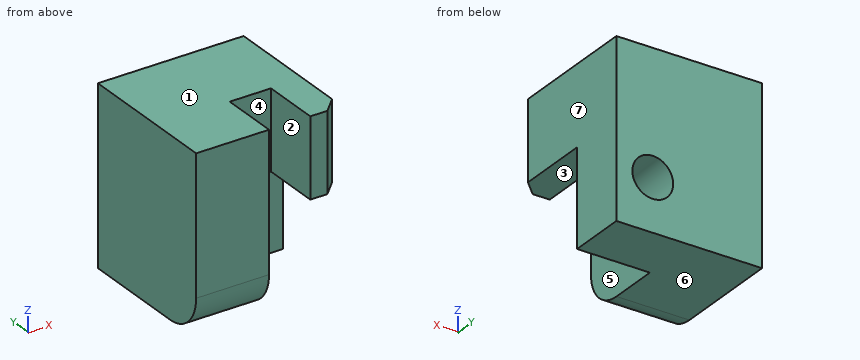
from build123d import *

# Parameters (mm, degrees)
F0_W     = 127
F0_H     = 152.4
F1_DEPTH = 127
F2_W     = 63.5
F2_H     = 83.7710094534
F3_DEPTH = 76.2
F4_R     = 17.78
F5_DEPTH = 50.8
F6_W     = 35.9447933733
F6_H     = 68.6289905466
F7_DEPTH = 50.8
F8_R     = 33.02
F9_SIZE  = 12.7


with BuildPart() as f1:
    # F0 (on Front) → F1 (new body)
    with BuildSketch(Plane.XZ):
        Rectangle(F0_W, F0_H)
    extrude(amount=F1_DEPTH)

    # F2 (on face) → F3 (cut)
    with BuildSketch(Plane.XZ.offset(127)):
        with Locations((31.75, -34.3144952733)):
            Rectangle(F2_W, F2_H)
    extrude(amount=-F3_DEPTH, mode=Mode.SUBTRACT)

    # F4 (on face) → F5 (cut, through all)
    with BuildSketch(Plane.XZ.offset(50.8)):
        with Locations((31.75, -30.5289905466)):
            Circle(F4_R)
    extrude(amount=-F5_DEPTH, mode=Mode.SUBTRACT)

    # F6 (on face) → F7 (cut)
    with BuildSketch(Plane.XZ.offset(127)):
        with Locations((17.9723966867, 41.8855047267)):
            Rectangle(F6_W, F6_H)
    extrude(amount=-F7_DEPTH, mode=Mode.SUBTRACT)

    # F8
    f8_edges = [f1.edges().sort_by_distance(p)[0] for p in [
        (-31.75, -127, -76.2),
    ]]
    fillet(f8_edges, radius=F8_R)

    # F9
    f9_edges = [f1.edges().sort_by_distance(p)[0] for p in [
        (63.5, -127, 41.885505),
    ]]
    chamfer(f9_edges, length=F9_SIZE)


solid = f1.part
CAD build for the part. Positions are in the model's coordinates, mm. Face numbers are marked on the shaded views. A direction names the side the tool comes from. Coordinates: 2 decimals unless noted, no trailing zeros. Write each loop counter-clockwise with the first axis right and the second up, starting at its lowest first coordinate (ties: lowest second). Pieces come first, ordered by that corner, then holes. Notation, with made-up numbers: M 66.25,72.25 L 98.25,72.25 A24 ccw 98.25,106.25 Z; hole C 89.25,-28 d5. An arc over 180 degrees is marked long. Answer as a JSON object with one key per item and string values. Group by question number.
1) Wall check: line 1 (Z direction, x = 31.75, y = -29.5); line 2 (X direction, y = -94, z = 29.5); line 3 (Y direction, x = 40, z = -9). Give the ranges that are in metal, low to high. Write a range as from..to.
2) Saw through at A-A (y = -89.5). Write the cut outline in (x, z).
3) Tool access for the marked faces 1, 2 and 3: list every direction of +Z, -Z, +X, -X, +Y, -Y with a clear straight run to the whole face (end or side of a thin tool).
4) Saw through at D-D (y = -72). Write the cut outline in (x, z), plus the area to 3 significant figures.
5) Mould opens along X. For the marked faces 4, 5, 6 and 7 say: +X half, -X half, draft (parallel to the pull), parting line (faces both ways), or undercut.
6) Saw through at B-B (x = 31.75). Write the cut outline in (y, z), plus the area to 3 significant figures.
7) Pin check, flat tips, straight feed: pin 1 Ø1.5 at (x, z) = (21.5, 56) entering from -Y; pin 2 Ø3 at (x, z) = (35.5, -60.5) entering from -Y. Stop position of each tip, or through.
8) Saw through at C-C (z = 19). Write the cut outline in (x, y), plus the area to 3 significant figures.
Values follow:
{
 "1": {"line 1": "z = -76.2..-48.31, -12.75..76.2", "line 2": "x = -63.5..0, 35.94..63.5", "line 3": "y = -50.8..0"},
 "2": {"outline": "M -63.5,-76.2 L 0,-76.2 L 0,76.2 L -63.5,76.2 Z; M 35.94,7.57 L 63.5,7.57 L 63.5,76.2 L 35.94,76.2 Z"},
 "3": {"face 1": "+Z, +X, -X, +Y, -Y", "face 2": "+Z, -Z, -Y", "face 3": "-Z, +X, -Y"},
 "4": {"outline": "M -63.5,-76.2 L 0,-76.2 L 0,7.57 L 63.5,7.57 L 63.5,76.2 L -63.5,76.2 Z", "area": "14,000 mm2"},
 "5": {"face 4": "undercut", "face 5": "undercut", "face 6": "draft", "face 7": "+X half"},
 "6": {"outline": "M -76.2,7.57 L -50.8,7.57 L -50.8,-12.75 L 0,-12.75 L 0,76.2 L -76.2,76.2 Z; M -50.8,-76.2 L 0,-76.2 L 0,-48.31 L -50.8,-48.31 Z", "area": "7,680 mm2"},
 "7": {"pin 1": "stops at y = -76.2", "pin 2": "stops at y = -50.8"},
 "8": {"outline": "M -63.5,-127 L 0,-127 L 0,-76.2 L 35.94,-76.2 L 35.94,-127 L 50.8,-127 L 63.5,-114.3 L 63.5,0 L -63.5,0 Z", "area": "14,200 mm2"}
}
